from build123d import *

# Parameters (mm, degrees)
BOSS_EXTRUDE1_DEPTH                            = 6.35
CUT_EXTRUDE1_DEPTH                             = 237.202948439
CUT_EXTRUDE2_DEPTH                             = 237.202948439
CUT_EXTRUDE3_DEPTH                             = 237.202948439
CUT_EXTRUDE4_DEPTH                             = 228.16972734
CSK_FOR_4_FLAT_HEAD_MACHINE_SCREW1_D           = 3.2639
CSK_FOR_4_FLAT_HEAD_MACHINE_SCREW1_CSINK_D     = 5.715
CSK_FOR_4_FLAT_HEAD_MACHINE_SCREW1_CSINK_ANGLE = 82
CSK_FOR_4_FLAT_HEAD_MACHINE_SCREW2_D           = 3.2639
CSK_FOR_4_FLAT_HEAD_MACHINE_SCREW2_CSINK_D     = 5.715
CSK_FOR_4_FLAT_HEAD_MACHINE_SCREW2_CSINK_ANGLE = 82
CSK_FOR_4_FLAT_HEAD_MACHINE_SCREW3_D           = 3.2639
CSK_FOR_4_FLAT_HEAD_MACHINE_SCREW3_CSINK_D     = 5.715
CSK_FOR_4_FLAT_HEAD_MACHINE_SCREW3_CSINK_ANGLE = 82


with BuildPart() as part:
    # Sketch1 → Boss-Extrude1 (new body)
    with BuildSketch(Plane(origin=(0, 0, 0), x_dir=(0, 0, -1), z_dir=(1, 0, 0))):
        Polygon((0, 0), (76.2, 131.982271537), (119.58608314, 131.982271537), (195.78608314, 0), (151.791992628, 0), (97.89304157, 93.355721707), (43.994090512, 0), align=None)
    extrude(amount=BOSS_EXTRUDE1_DEPTH)

    # Sketch2 → Cut-Extrude1 (cut, through all)
    with BuildSketch(Plane(origin=(6.35, 0, 0), x_dir=(0, 0, -1), z_dir=(1, 0, 0))):
        Polygon((43.994090512, 0), (10.998522628, 19.05), (0, 0), align=None)
    extrude(amount=-CUT_EXTRUDE1_DEPTH, mode=Mode.SUBTRACT)

    # Sketch3 → Cut-Extrude2 (cut, through all)
    with BuildSketch(Plane(origin=(6.35, 0, 0), x_dir=(0, 0, -1), z_dir=(1, 0, 0))):
        Polygon((43.994090512, 0), (31.620752556, 7.14375), (41.145752556, 23.641533942), (53.519090512, 16.497783942), align=None)
    extrude(amount=-CUT_EXTRUDE2_DEPTH, mode=Mode.SUBTRACT)

    # Sketch4 → Cut-Extrude3 (cut, through all)
    with BuildSketch(Plane(origin=(6.35, 0, 0), x_dir=(0, 0, -1), z_dir=(1, 0, 0))):
        Polygon((151.791992628, 0), (184.787560512, 19.05), (195.78608314, 0), align=None)
    extrude(amount=-CUT_EXTRUDE3_DEPTH, mode=Mode.SUBTRACT)

    # Sketch5 → Cut-Extrude4 (cut, through all)
    with BuildSketch(Plane(origin=(6.35, 0, 0), x_dir=(0, 0, -1), z_dir=(1, 0, 0))):
        Polygon((151.791992628, 0), (164.165330584, 7.14375), (154.640330584, 23.641533942), (142.266992628, 16.497783942), align=None)
    extrude(amount=-CUT_EXTRUDE4_DEPTH, mode=Mode.SUBTRACT)

    # CSK for #4 Flat Head Machine Screw1 (through all)
    with Locations(Plane.ZY):
        with Locations((-161.803140841, 23.935182653)):
            CounterSinkHole(CSK_FOR_4_FLAT_HEAD_MACHINE_SCREW1_D / 2, CSK_FOR_4_FLAT_HEAD_MACHINE_SCREW1_CSINK_D / 2, counter_sink_angle=CSK_FOR_4_FLAT_HEAD_MACHINE_SCREW1_CSINK_ANGLE)

    # CSK for #4 Flat Head Machine Screw2 (through all)
    with Locations(Plane.ZY):
        with Locations((-158.628140841, 29.434443967)):
            CounterSinkHole(CSK_FOR_4_FLAT_HEAD_MACHINE_SCREW2_D / 2, CSK_FOR_4_FLAT_HEAD_MACHINE_SCREW2_CSINK_D / 2, counter_sink_angle=CSK_FOR_4_FLAT_HEAD_MACHINE_SCREW2_CSINK_ANGLE)

    # CSK for #4 Flat Head Machine Screw3 (through all)
    with Locations(Plane.ZY):
        with Locations((-37.157942299, 29.434443967), (-33.982942299, 23.935182653)):
            CounterSinkHole(CSK_FOR_4_FLAT_HEAD_MACHINE_SCREW3_D / 2, CSK_FOR_4_FLAT_HEAD_MACHINE_SCREW3_CSINK_D / 2, counter_sink_angle=CSK_FOR_4_FLAT_HEAD_MACHINE_SCREW3_CSINK_ANGLE)


solid = part.part
Input: part model. Units: mm. Frame: model coordinates. A direction names the side the tool comes from. Coordinates: 2 decimals unless noted, no trailing zeros. Loops run counter-clockwise (first coordinate to the right, second up) from the corner with the lowest first, then second, coordinate; pieces in that order, holes last. Notation, with made-up numbers: (-33.75, 82) - (-15.75, 82) arc R31 ccw to (-15.75, 112) - close; hole circle Ø7 at (62, -37.5). An arc over 180 degrees is marked (long way). Answer in a Markdown table with one row per item. Add a question column.
Item 1: Access query for faces 4 (the flat face through (3.22, 20.12, -148.54)), 5 (the flat face through (3.131, 74.726, -43.143)). Directions: +Z, -Z, +X, -X, +Y, -Y. A direction counts if a zero-diameter tool reaches every point of the face in a straight line with its end or side. Return the directions, or none.
Item 2: Section query C-C on z = -166.5. Return the cut outline in (x, y).
Item 3: Mould query, pull axis Y, two halves, no side actions, for faces 1 (the flat face through (3, 131.982, -98)), 2 (the cylindrical face through (3.91, 23.31, -35.49)), 3 (the flat face through (3.22, 15.28, -36.32)). Classes: released by +Y, released by -Y, zero draft, split by the parting line, or undercut.
Item 4: Section query D-D on y = 122.5. Return the cut outline in (x, z).
Item 5: Line query: line 1 along Z through (x, y) = (1, 29.5); line 2 along Z through (x, y) = (5.5, 60.5); line 3 along Z through (x, y) = (2.5, 55). Output: solid intervals per line, ascending. Write a range as [from, to].
Item 6: Contact query for flat-ended pins moving along their axis: P1, Ø3, axis at x = 4.5, z = -134, coming from the -Y side; P2, Ø2, axis at y = 23.94, z = -161.8, coming from the -X side (3 decimals); P3, Ø4, axis at y = 29.43, z = -37.16, coming from the -X side; P4, Ø2, axis at x = 3.5, y = 94.5, coming from the -Z side. Output: stop coordinate, or through.
Item 7: Section query B-B on x = 3.5. Return the cut outline in (y, z).
Item 8: Section query A-A on y = 88. Return the cut outline in (x, z).
Recorded:
| question | item | result |
|---|---|---|
| 1 | face 4 | +X, -X, -Y |
| 1 | face 5 | +Z, +X, -X, +Y |
| 2 | outline | (0, 8.49) - (6.35, 8.49) - (6.35, 50.72) - (0, 50.72) - close |
| 3 | face 1 | released by +Y |
| 3 | face 2 | undercut |
| 3 | face 3 | released by -Y |
| 4 | outline | (0, -125.06) - (6.35, -125.06) - (6.35, -70.73) - (0, -70.73) - close |
| 5 | line 1 | [-178.75, -160.62], [-156.64, -134.76], [-61.03, -39.15], [-35.17, -17.03] |
| 5 | line 2 | [-160.86, -116.86], [-78.92, -34.93] |
| 5 | line 3 | [-164.03, -120.04], [-75.75, -31.75] |
| 6 | P1 | y = 28.22 |
| 6 | P2 | through |
| 6 | P3 | x = 0.98 |
| 6 | P4 | z = -141.8 |
| 7 | outline | (7.14, -164.17) - (19.05, -184.79) - (131.98, -119.59) - (131.98, -76.2) - (19.05, -11) - (7.14, -31.62) - (23.64, -41.15) - (16.5, -53.52) - (93.36, -97.89) - (16.5, -142.27) - (23.64, -154.64) - close; hole circle Ø3.26 at (23.94, -161.8); hole circle Ø3.26 at (23.94, -33.98); hole circle Ø3.26 at (29.43, -158.63); hole circle Ø3.26 at (29.43, -37.16) |
| 8 | outline | (0, -144.98) - (6.35, -144.98) - (6.35, -100.99) - (0, -100.99) - close; (0, -94.8) - (6.35, -94.8) - (6.35, -50.81) - (0, -50.81) - close |
